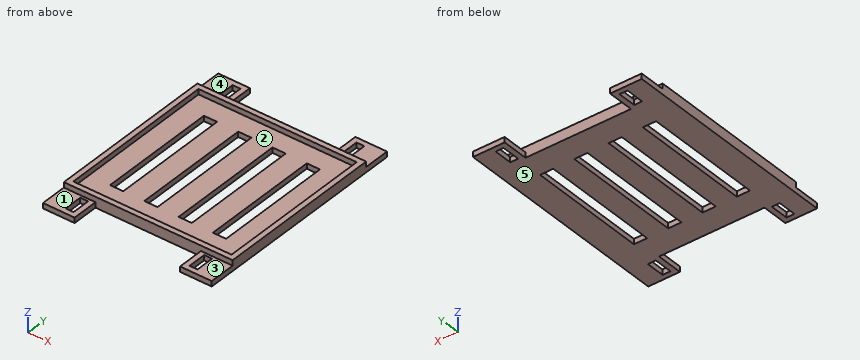
```python
from build123d import *

# Parameters (mm, degrees)
SKETCH_W      = 5
SKETCH_H      = 45
SKETCH_W_2    = 3
SKETCH_H_2    = 7
PAD_DEPTH     = 2
SKETCH006_W   = 64
SKETCH006_H   = 64
SKETCH006_W_2 = 60
SKETCH006_H_2 = 60
PAD001_DEPTH  = 2


with BuildPart() as part:
    # Sketch → Pad (new body)
    with BuildSketch(Plane.XY):
        Polygon((64, 0), (64, 84), (52, 84), (52, 74), (12, 74), (12, 84), (0, 84), (0, 0), (12, 0), (12, 10), (52, 10), (52, 0), align=None)
        with Locations((12.5, 42)):
            Rectangle(SKETCH_W, SKETCH_H, mode=Mode.SUBTRACT)
        with Locations((25.5, 42)):
            Rectangle(SKETCH_W, SKETCH_H, mode=Mode.SUBTRACT)
        with Locations((38.5, 42)):
            Rectangle(SKETCH_W, SKETCH_H, mode=Mode.SUBTRACT)
        with Locations((51.5, 42)):
            Rectangle(SKETCH_W, SKETCH_H, mode=Mode.SUBTRACT)
        with Locations((8.5, 78.5)):
            Rectangle(SKETCH_W_2, SKETCH_H_2, mode=Mode.SUBTRACT)
        with Locations((55.5, 78.5)):
            Rectangle(SKETCH_W_2, SKETCH_H_2, mode=Mode.SUBTRACT)
        with Locations((55.5, 5.5)):
            Rectangle(SKETCH_W_2, SKETCH_H_2, mode=Mode.SUBTRACT)
        with Locations((8.5, 5.5)):
            Rectangle(SKETCH_W_2, SKETCH_H_2, mode=Mode.SUBTRACT)
    extrude(amount=PAD_DEPTH)

    # Sketch006 → Pad001 (join)
    with BuildSketch(Plane.XY.offset(2)):
        with Locations((32, 42)):
            Rectangle(SKETCH006_W, SKETCH006_H)
        with Locations((32, 42)):
            Rectangle(SKETCH006_W_2, SKETCH006_H_2, mode=Mode.SUBTRACT)
    extrude(amount=PAD001_DEPTH)


solid = part.part
```
Here's how the part is built. I have some questions about the finished solid (model axes, mm). Face numbers are marked on the shaded views. A direction names the side the tool comes from. Give positions to 0.01 mm unless a question says otherwise; leave off trailing zeros. Loops run counter-clockwise (first coordinate to the right, second up) from the corner with the lowest first, then second, coordinate; pieces in that order, holes last. Notation, with made-up numbers: M -21,43 L -6,43 A16 cw -6,63 Z; hole C -29,71.25 d10. An arc over 180 degrees is marked long. Return JSON: item names as keys, results as strings.
Item 1: Imagine slicing it at A-A on y = 58. List the corners of the cut face in (x, z) for me.
A:
{"outline": "M 0,0 L 10,0 L 10,2 L 2,2 L 2,4 L 0,4 Z; M 15,0 L 23,0 L 23,2 L 15,2 Z; M 28,0 L 36,0 L 36,2 L 28,2 Z; M 41,0 L 49,0 L 49,2 L 41,2 Z; M 54,0 L 64,0 L 64,4 L 62,4 L 62,2 L 54,2 Z"}
Item 2: Imagine slicing it at B-B on x = 17. List the corners of the cut face in (y, z) for me, then the cut area to 3 significant figures.
A:
{"outline": "M 10,0 L 74,0 L 74,4 L 72,4 L 72,2 L 12,2 L 12,4 L 10,4 Z", "area": "136 mm^2"}
Item 3: Please list where these lines run through material, in increasing order: line 1 (X direction, y = 23.5, z = 1.25); line 2 (X direction, y = 6, z = 0.7); line 3 (Y direction, x = 15.5, z = 3.7).
A:
{"line 1": "x = 0 to 10, 15 to 23, 28 to 36, 41 to 49, 54 to 64", "line 2": "x = 0 to 7, 10 to 12, 52 to 54, 57 to 64", "line 3": "y = 10 to 12, 72 to 74"}
Item 4: Imagine slicing it at C-C on z = 1. State how many separate pieces and enclosed holes the cut face has, then the cut area to 3 significant figures.
A:
{"separate pieces": "1", "enclosed holes": "8", "area": "3,590 mm^2"}
Item 5: Imagine slicing it at D-D on x = 6. List the corners of the cut face in (y, z) for me.
A:
{"outline": "M 0,0 L 84,0 L 84,2 L 74,2 L 74,4 L 72,4 L 72,2 L 12,2 L 12,4 L 10,4 L 10,2 L 0,2 Z"}
Item 6: Thinking about a two-plate mould opening in X: for the marked faces 1 and 2, which applies, released by +X, released by -X, zero draft, split by the parting line, or undercut?
A:
{"face 1": "zero draft", "face 2": "undercut"}
Item 7: I'm going to push flat-ended pins straight in: pin 1 Ø5 at (x, y) = (4, 80) entering from +Z; pin 2 Ø1.6 at (x, z) = (21, 3) entering from +Y; pin 3 Ø1 at (x, z) = (29, 1) entering from -Y. Where does each tip first touch, or does it pass through?
A:
{"pin 1": "stops at z = 2", "pin 2": "stops at y = 74", "pin 3": "stops at y = 10"}
Item 8: On a 3-axis mill with a long thin cutter (end or side, diameter ignored), from which of +Z, -Z, +X, -X, +Y, -Y can I reach the whole of each face in a straight line? I mean the marked faces 3, 4 and 5. Say none if no direction works.
A:
{"face 3": "+Z, +X, -X, -Y", "face 4": "+Z, +X, -X, +Y", "face 5": "-Z, +X, -X, +Y, -Y"}
